from build123d import *

# Parameters (mm, degrees)
F0_W      = 254
F0_H      = 127
F1_DEPTH  = 228.6
F3_DEPTH  = 1270
F5_DEPTH  = 38.1
F6_W      = 104.14
F6_H      = 25.4
F7_DEPTH  = 127
F8_R      = 15.24
F9_DEPTH  = 1270
F10_W     = 76.2
F10_H     = 20.32
F11_DEPTH = 1270


with BuildPart() as f1:
    # F0 (on Front) → F1 (new body)
    with BuildSketch(Plane.XZ):
        Rectangle(F0_W, F0_H)
    extrude(amount=-F1_DEPTH)

    # F2 (on face) → F3 (cut)
    with BuildSketch(Plane.XZ):
        Polygon((127, 63.5), (15.24, 63.5), (127, -63.5), align=None)
    extrude(amount=-F3_DEPTH, mode=Mode.SUBTRACT)

    # F4 (on face) → F5 (cut)
    with BuildSketch(Plane.XZ):
        Polygon((50.8, -63.5), (127, -63.5), (50.8, 23.0909090909), align=None)
    extrude(amount=-F5_DEPTH, mode=Mode.SUBTRACT)

    # F6 (on face) → F7 (cut)
    with BuildSketch(Plane.XZ):
        with Locations((-74.93, -50.8)):
            Rectangle(F6_W, F6_H)
    extrude(amount=-F7_DEPTH, mode=Mode.SUBTRACT)

    # F8 (on face) → F9 (cut)
    with BuildSketch(Plane(origin=(40.081154193, 0, 35.2714156898), x_dir=(0, 1, 0), z_dir=(0.7507135169, 0, 0.6606278949))):
        with Locations((76.2, -31.4652394879)):
            Circle(F8_R)
        with Locations((190.5, -31.4652394879)):
            Circle(F8_R)
        with Locations((190.5, -93.4700509759)):
            Circle(F8_R)
        with Locations((76.2, -93.4700509759)):
            Circle(F8_R)
    extrude(amount=-F9_DEPTH, mode=Mode.SUBTRACT)

    # F10 (on face) → F11 (cut)
    with BuildSketch(Plane(origin=(-127, 0, 0), x_dir=(0, -1, 0), z_dir=(-1, 0, 0))):
        with Locations((-114.3, 53.34)):
            Rectangle(F10_W, F10_H)
    extrude(amount=-F11_DEPTH, mode=Mode.SUBTRACT)


solid = f1.part
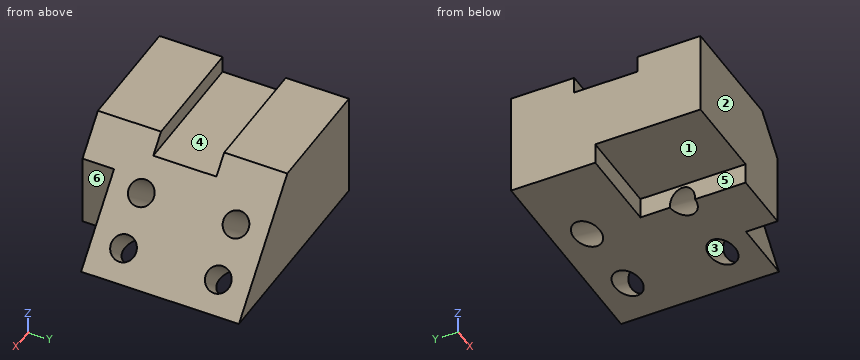
Read the model definition and answer for the solid it produces. Units are mm, in the model's axes. Face numbers are marked on the shaded views. A direction names the side the tool comes from. Give positions to 0.01 mm unless a question says otherwise; leave off trailing zeros. Loops run counter-clockwise (first coordinate to the right, second up) from the corner with the lowest first, then second, coordinate; pieces in that order, holes last. Notation, with made-up numbers: M 73,78 L 81,78 A26 ccw 81,115 Z; hole C -27.75,79 d1. An arc over 180 degrees is marked long. Write each question's results on one line, items separated by ' | '.
1. Section B-B on y = 110.5 is taken. Give the vertices of the cut face in (x, z), plus the area to 3 significant figures.
Values:
outline: M -127,-38.1 L -22.86,-38.1 L -22.86,-63.5 L 127,-63.5 L 33.12,43.18 L -127,43.18 Z | area: 19,400 mm^2
2. The mould has two halves that part along Y. Classify the marked faces 1, 2 and 3: pulls with the +Y half, pulls with the -Y half, needs draft (parallel to the pull), parting line crosses it, or undercut.
Values:
face 1: needs draft | face 2: pulls with the -Y half | face 3: undercut
3. Straight lines are drawn through the part: line 1 (Y direction, x = -41, z = 50); line 2 (Y direction, x = 17, z = -32.5); line 3 (Z direction, x = -79, y = 101.5). For each, find the intervals that lie inside material, in ascending order. Write a range as [from, to].
Values:
line 1: y = [0, 76.2], [152.4, 228.6] | line 2: y = [0, 61.54], [90.86, 175.84], [205.16, 228.6] | line 3: z = [-38.1, 43.18]
4. A tool of negligible diameter and unlimited length cuts with its end or side. For the marked faces 4, 5 and 6, from which of +Z, -Z, +X, -X, +Y, -Y can it reach the whole face along a straight path? Write none if from no direction.
Values:
face 4: +Z, +X, -X | face 5: -Z, -X, -Y | face 6: +Z, -Z, +X, -Y
5. Section A-A on x = -100.5 is taken. Give the vertices of the cut face in (y, z).
Values:
outline: M 0,-38.1 L 127,-38.1 L 127,-63.5 L 228.6,-63.5 L 228.6,63.5 L 152.4,63.5 L 152.4,43.18 L 76.2,43.18 L 76.2,63.5 L 0,63.5 Z
6. Given pin 1 (5 mm diameter, centred on x = -27.5, y = 126, fed in from +Z); pin 2 (1.5 mm diameter, centred on y = 57, z = 19.5, fed in from +X); pin 3 (12 mm diameter, centred on y = 87.5, z = 15.5, fed in from +X), each flat-ended and moving along its own axis, determine where each tip first touches the part or whether it passes through.
Values:
pin 1: stops at z = 43.18 | pin 2: stops at x = 54.62 | pin 3: stops at x = 61.48
7. Section D-D on z = -48 is taken. State how many separate pieces and enclosed holes the cut face has, plus the area to 3 significant figures.
Values:
separate pieces: 1 | enclosed holes: 3 | area: 35,000 mm^2
8. Section C-C on z = 29 is taken. Give the vertices of the cut face in (x, y).
Values:
outline: M -127,0 L 45.6,0 L 45.6,228.6 L -127,228.6 Z
